Check sheet for the modelled part. Datum: model origin and axes. Units: mm. A direction names the side the tool comes from. Give positions to 0.01 mm unless a question says otherwise; leave off trailing zeros. Order: outer loops, then holes, each group sorted by start corner. A loop starts at its lowest first (then second) coordinate and runs counter-clockwise, first axis right, second up.
```python
from build123d import *

# Parameters (mm, degrees)
F1_DEPTH = 14.224


with BuildPart() as f1:
    # F0 (on Top) → F1 (new body)
    with BuildSketch(Plane.XY):
        with BuildLine():
            Line((-10.127848, 43.296553), (-9.115064, 59.754308))
            Line((-9.115064, 59.754308), (-32.915507, 62.033072))
            Line((-32.915507, 62.033072), (-59.501108, 59.501108))
            ThreePointArc((-59.501108, 59.501108), (-55.542844, 57.573082), (-55.449966, 53.171206))
            Line((-55.449966, 53.171206), (-55.449966, 36.713451))
            ThreePointArc((-55.449966, 36.713451), (-60.387293, 35.617261), (-65.324619, 36.713451))
            ThreePointArc((-65.324619, 36.713451), (-63.738246, 29.492092), (-67.350194, 23.040855))
            ThreePointArc((-67.350194, 23.040855), (-61.40008, 24.486692), (-55.449966, 23.040855))
            Line((-55.449966, 23.040855), (-55.449966, 5.823513))
            ThreePointArc((-55.449966, 5.823513), (-57.376818, 0.42562), (-62.286269, -2.531962))
            Line((-62.286269, -2.531962), (-34.941077, -2.531962))
            ThreePointArc((-34.941077, -2.531962), (-39.686396, -0.513738), (-41.524179, 4.304335))
            Line((-41.524179, 4.304335), (-41.524179, 23.294052))
            Line((-41.524179, 23.294052), (-27.851583, 23.294052))
            Line((-27.851583, 23.294052), (-27.851583, 10.634242))
            ThreePointArc((-27.851583, 10.634242), (-20.962224, 2.533472), (-10.63424, 0))
            Line((-10.63424, 0), (6.329905, -4.304335))
            Line((6.329905, -4.304335), (6.329905, -13.925791))
            Line((6.329905, -13.925791), (-10.63424, -13.925791))
            ThreePointArc((-10.63424, -13.925791), (-18.964741, -12.696939), (-26.585601, -9.115064))
            Line((-26.585601, -9.115064), (-26.585601, -25.319621))
            ThreePointArc((-26.585601, -25.319621), (-10.325346, -27.500204), (6.076708, -27.851582))
            Line((6.076708, -27.851582), (6.076708, -55.19677))
            Line((6.076708, -55.19677), (58.741521, -53.171206))
            ThreePointArc((58.741521, -53.171206), (53.457994, -49.925807), (54.437183, -43.802943))
            Line((54.437183, -43.802943), (52.411616, 8.861868))
            Line((52.411616, 8.861868), (35.707628, 9.202845))
            ThreePointArc((35.707628, 9.202845), (40.89498, 6.062472), (40.764589, 0))
            Line((40.764589, 0), (40.764589, -41.270979))
            Line((40.764589, -41.270979), (21.530654, -42.010745))
            Line((21.530654, -42.010745), (20.16781, -6.576743))
            ThreePointArc((20.16781, -6.576743), (19.622446, 2.526197), (12.406613, 8.102279))
            Line((12.406613, 8.102279), (-13.558293, 14.219645))
            Line((-13.558293, 14.219645), (-13.558293, 23.040855))
            Line((-13.558293, 23.040855), (5.570316, 23.040855))
            ThreePointArc((5.570316, 23.040855), (9.494858, 24.410603), (13.419399, 23.040855))
            Line((13.419399, 23.040855), (21.26848, 27.598385))
            Line((21.26848, 27.598385), (29.623957, 30.130347))
            ThreePointArc((29.623957, 30.130347), (21.62589, 33.222018), (14.178989, 37.473038))
            ThreePointArc((14.178989, 37.473038), (12.02682, 35.606476), (9.874651, 37.473038))
            Line((9.874651, 37.473038), (-42.030569, 37.473038))
            Line((-42.030569, 37.473038), (-42.030569, 47.854081))
            Line((-42.030569, 47.854081), (-22.281267, 47.854081))
            ThreePointArc((-22.281267, 47.854081), (-15.791339, 46.677234), (-10.127848, 43.296553))
        make_face()
    extrude(amount=F1_DEPTH)


solid = f1.part
```
(1) Release check for a two-part mould opening along X. For faces 5 (the face through (-35, 23.294, 7)), 6 (the face through (-49, -2.532, 7)), 7 (the face through (40.85, 6.14, 7.01)), 8 (the face through (25.388, 28.847, 7.012)) record: released by +X, released by -X, zero draft, split by the parting line, or undercut.
Response values:
face 5: undercut
face 6: zero draft
face 7: undercut
face 8: released by +X
(2) Set-up check for faces 1 (the face through (-4, 23.041, 7)), 2 (the face through (-26.586, -17, 7)), 3 (the face through (-0.394, 11.118, 7.012)), 4 (the face through (-20.849, 60.878, 7.012)): record each of +Z, -Z, +X, -X, +Y, -Y from which the full face is reachable in a straight line by a thin tool's end or side.
Response values:
face 1: +Z, -Z, +X
face 2: +Z, -Z, -X, -Y
face 3: +Z, -Z
face 4: +Z, -Z, +X, +Y
(3) Cross-section at D-D on y = 55.5. Enter the section's corners in (x, z), then the cut area to 3 significant figures.
Response values:
outline: (-54.88, 0) - (-9.38, 0) - (-9.38, 14.22) - (-54.88, 14.22) - close
area: 647 mm2
(4) Cross-section at C-C on x = -2. Enter the section's corners in (y, z), then the cut area to 3 significant figures.
Response values:
outline: (-27.91, 0) - (-13.93, 0) - (-13.93, 14.22) - (-27.91, 14.22) - close; (-2.19, 0) - (11.5, 0) - (11.5, 14.22) - (-2.19, 14.22) - close; (23.04, 0) - (37.47, 0) - (37.47, 14.22) - (23.04, 14.22) - close
area: 599 mm2
(5) Cross-section at A-A on y = -35. Enter the section's corners in (x, z), then the cut area to 3 significant figures.
Response values:
outline: (6.08, 0) - (21.26, 0) - (21.26, 14.22) - (6.08, 14.22) - close; (40.76, 0) - (54.1, 0) - (54.1, 14.22) - (40.76, 14.22) - close
area: 406 mm2
(6) Material ranges on L1, parallel to X at y = 21.5, z = 7.5; L2, parallel to Y at x = -22.5, z = 7.25; L3, parallel to Y at x = -26, z = 11.75, recorded low to high.
Response values:
L1: x = -55.45 to -41.52, -27.85 to -13.56
L2: y = -26.04 to -11.37, 3.6 to 37.47, 47.85 to 61.04
L3: y = -25.43 to -9.49, 7.27 to 37.47, 47.85 to 61.37
(7) Cross-section at B-B on x = -30. Enter the section's corners in (y, z), then the cut area to 3 significant figures.
Response values:
outline: (23.29, 0) - (37.47, 0) - (37.47, 14.22) - (23.29, 14.22) - close; (47.85, 0) - (61.75, 0) - (61.75, 14.22) - (47.85, 14.22) - close
area: 399 mm2
(8) Gauge pin test, flat ends, axial feed: pin 1 Ø1 at (y, z) = (-34, 5) entering from -X; pin 2 Ø2 at (y, z) = (25, 12.5) entering from +X; pin 3 Ø4.5 at (x, z) = (0.5, 5) entering from -Y. Record the tip position at first contact, or that the pin passes through.
Response values:
pin 1: stops at x = 6.08
pin 2: stops at x = 18.52
pin 3: stops at y = -27.94
